```python
from build123d import *

# Parameters (mm, degrees)
F1_DEPTH     = 4.318
F1_FACE_W    = 8.4660017827
F1_FACE_H    = 4.318
F4_W         = 8.4660017827
F4_H         = 4.318
F5_DEPTH     = 0.508
F7_DEPTH     = 13.462
F9_T1_DEPTH  = 101.8009504956
F10_T1_DEPTH = 101.8156278686
F8_FACE_W    = 35.3900017827
F8_FACE_H    = 4.318
F14_DEPTH    = 45.466


# Not quite as in the source:
# - a fillet or chamfer that OpenCascade refuses, or shapes differently, is made with other operations: its cross-section is extruded or revolved along the edge and cut away or added


with BuildPart() as f1:
    # F0 (on Front) → F1 (new body)
    with BuildSketch(Plane.XZ):
        with BuildLine():
            ThreePointArc((-14.8547158409, -68.6793103814), (-12.973951869, -74.217922925), (-7.62, -76.5734910965))
            Line((-7.62, -76.5734910965), (7.62, -76.5734910965))
            ThreePointArc((7.62, -76.5734910965), (12.9819628095, -74.2196084737), (14.8784083325, -68.6793103814))
            Line((14.8784083325, -68.6793103814), (14.8547158409, -68.6793103814))
            Line((14.8547158409, -68.6793103814), (-14.8547158409, -68.6793103814))
        make_face()
        Polygon((-7.1831139455, 19.1512540919), (-14.8547158409, -68.6793103814), (14.8547158409, -68.6793103814), (7.1831139455, 19.1512540919), (4.2330008913, 52.9264810056), (-4.2330008913, 52.9264810056), align=None)
    extrude(amount=F1_DEPTH)

    # F3: sweep along a path in F2
    with BuildLine(Plane.YZ) as f3_path:
        Line((-4.318, 52.9264810056), (-4.318, 55.3578620488))
        ThreePointArc((-4.318, 55.3578620488), (-3.7519884271, 59.1070386053), (-2.1044055351, 62.5220297571))
        ThreePointArc((-2.1044055351, 62.5220297571), (2.3667917296, 72.1058812805), (3.5367051605, 82.6165005565))
    # F1_face (on face) → F3 (sweep)
    with BuildSketch(Plane(origin=(0, -2.159, 52.9264810056), x_dir=(1, 0, 0), z_dir=(0, 0, 1))):
        Rectangle(F1_FACE_W, F1_FACE_H)
    sweep(path=f3_path.line)

    # F4 (on face) → F5 (join)
    with BuildSketch(Plane(origin=(0, -4.2773000259, 82.2099457989), x_dir=(1, 0, 0), z_dir=(0, -0.0519587059, 0.9986492342))):
        with Locations((0, 9.9835743541)):
            Rectangle(F4_W, F4_H)
    extrude(amount=F5_DEPTH)

    # F6 (on face) → F7 (join)
    with BuildSketch(Plane.YZ.offset(4.2330008913)):
        with BuildLine():
            Line((-4.318, 52.9264810056), (0, 52.9264810056))
            Line((0, 52.9264810056), (0, 55.3578620488))
            ThreePointArc((0, 55.3578620488), (0.3735676381, 57.8323185761), (1.4609723468, 60.0862127363))
            ThreePointArc((1.4609723468, 60.0862127363), (6.5240819847, 70.938807275), (7.8488725536, 82.8408582485))
            Line((7.8488725536, 82.8408582485), (7.822477531, 83.3481720595))
            Line((7.822477531, 83.3481720595), (3.5103101379, 83.1238143674))
            Line((3.5103101379, 83.1238143674), (3.5367051605, 82.6165005565))
            ThreePointArc((3.5367051605, 82.6165005565), (2.3667917296, 72.1058812805), (-2.1044055351, 62.5220297571))
            ThreePointArc((-2.1044055351, 62.5220297571), (-3.7519884271, 59.1070386053), (-4.318, 55.3578620488))
            Line((-4.318, 55.3578620488), (-4.318, 52.9264810056))
        make_face()
    extrude(amount=F7_DEPTH)

    # F8: F1 across plane


with BuildPart() as f1_1:
    add(f1.part)
    add(f1.part.mirror(Plane.YZ))

    # F9: fillet of radius 20.8491483247 on 1 edges, made by hand

    # F9_s2 → F9_t1 (cut)
    with BuildSketch(Plane.XZ.offset(-48.7414752478)):
        with BuildLine():
            ThreePointArc((17.6950008913, 72.4230711047), (14.0025238199, 60.5767376056), (4.2330008913, 52.9264810056))
            Line((4.2330008913, 52.9264810056), (17.6950008913, 52.9264810056))
            Line((17.6950008913, 52.9264810056), (17.6950008913, 72.4230711047))
        make_face()
    extrude(amount=F9_T1_DEPTH, mode=Mode.SUBTRACT)

    # F10: fillet of radius 20.8534 on 1 edges, made by hand

    # F10_s2 → F10_t1 (cut)
    with BuildSketch(Plane.XZ.offset(-48.7488139343)):
        with BuildLine():
            ThreePointArc((-4.2330008913, 52.9264810056), (-14.0026048293, 60.5784652564), (-17.6950008913, 72.4260065793))
            Line((-17.6950008913, 72.4260065793), (-17.6950008913, 52.9264810056))
            Line((-17.6950008913, 52.9264810056), (-4.2330008913, 52.9264810056))
        make_face()
    extrude(amount=F10_T1_DEPTH, mode=Mode.SUBTRACT)

    # F12: sweep along a path in F11
    with BuildLine(Plane.YZ) as f12_path:
        ThreePointArc((5.6663938345, 83.2359932134), (4.2906494395, 90.7738508992), (1.2476332355, 97.8060641719))
        Line((1.2476332355, 97.8060641719), (-17.8702931298, 131.016411811))
    # F8_face (on face) → F12 (sweep)
    with BuildSketch(Plane(origin=(0, 5.6663938345, 83.2359932134), x_dir=(1, 0, 0), z_dir=(0, -0.0519587059, 0.9986492342))):
        Rectangle(F8_FACE_W, F8_FACE_H)
    sweep(path=f12_path.line)

    # F13 (on face) → F14 (cut)
    with BuildSketch(Plane(origin=(0, 41.3553334691, 23.8066830455), x_dir=(1, 0, 0), z_dir=(0, -0.8666583712, -0.4989020622))):
        Polygon((-6.7998209327, 122.4935306315), (-14.8516167313, 122.4935306315), (-11.232118832, 81.1224803329), (-10.419318832, 81.1224803329), align=None)
        Polygon((4.0258978993, 122.4935306315), (-4.0258978993, 122.4935306315), (-0.4064, 81.1224803329), (0, 81.1224803329), (0.4064, 81.1224803329), align=None)
        Polygon((11.232118832, 81.1224803329), (14.8516167313, 122.4935306315), (6.7998209327, 122.4935306315), (10.419318832, 81.1224803329), align=None)
    extrude(amount=-F14_DEPTH, mode=Mode.SUBTRACT)


solid = f1_1.part
```
CAD build for the part. Positions are in the model's coordinates, mm. A direction names the side the tool comes from. Round coordinates to 2 decimals unless told otherwise and drop trailing zeros. Order: outer loops, then holes, each group sorted by start corner. A loop starts at its lowest first (then second) coordinate and runs counter-clockwise, first axis right, second up. Notation, with made-up numbers: (19.5, 5) - (52.5, 5) arc R12 cw to (52.5, 10) - close; hole circle Ø4 at (89, 89.25). An arc over 180 degrees is marked (long way). Answer in a Markdown table with one row per item. Add a question column.
(1) Mould opens along X. For faces 1 (the face through (-8.635, -7.448, 112.85)), 2 (the face through (-12.925, -2.129, -74.281)), 3 (the face through (-15.329, -8.208, 109.904)) say: +X half, -X half, draft (parallel to the pull), parting line (faces both ways), or undercut.
(2) Probe L1, parallel to Y at x = -2, z = 38.5; L2, parallel to Z at x = 3, y = -2.25; L3, parallel to X at y = -1.75, z = -19. List the from-to ranges inside material, lowest first. Write a range as [from, to].
(3) Band-saw the part on B-B on y = -6.25. List the corners of the cut face in (x, z) (3 decimals).
(4) Band-saw the part on C-C on z = 67. List the corners of the cut face in (x, y), and give its area (3 significant figures).
(5) Band-saw the part on A-A on z = 107. List the corners of the cut face in (x, y) (3 decimals).
(6) Band-saw the part on D-D on z = -40. List the corners of the cut face in (x, y).
(7) Drop flat-ended pins along their axis: pin 1 Ø12 at (x, y) = (3.5, -4) entering from +Z; pin 2 Ø8 at (x, z) = (13.5, 18.5) entering from +Y; pin 3 Ø4 at (y, z) = (-3.5, -33) entering from -X; pin 4 Ø4 at (y, z) = (2.5, 69) entering from +X. Give the stop position or say it passes through.
(8) 3-axis set-ups, long thin cutter, end or side, ignore diameter. For faces 4 (the face through (14.1, 0.13, 60.72)), 5 (the face through (0, 0, -26)), 6 (the face through (15.242, -8.208, 109.904)): which of +Z, -Z, +X, -X, +Y, -Y reach the whole face in a straight line?
Data:
| question | item | result |
|---|---|---|
| 1 | face 1 | undercut |
| 1 | face 2 | -X half |
| 1 | face 3 | draft |
| 2 | L1 | y = [-4.32, 0] |
| 2 | L2 | z = [-76.57, 62.3], [99.55, 108.21] |
| 2 | L3 | x = [-10.52, 10.52] |
| 3 | outline | (-17.695, 106.503) - (-12.483, 106.503) - (-13.139, 115.157) - (-17.695, 115.157) - close; (-9.168, 106.503) - (-1.657, 106.503) - (-2.313, 115.157) - (-8.512, 115.157) - close; (1.657, 106.503) - (9.168, 106.503) - (8.512, 115.157) - (2.313, 115.157) - close; (12.483, 106.503) - (17.695, 106.503) - (17.695, 115.157) - (13.139, 115.157) - close |
| 4 | outline | (-16.98, 0.46) - (16.98, 0.46) - (16.98, 5.17) - (-16.98, 5.17) - close |
| 4 | area | 160 mm^2 |
| 5 | outline | (-17.695, -6.536) - (-12.533, -6.536) - (-12.316, -1.554) - (-17.695, -1.554) - close; (-9.336, -1.554) - (-9.118, -6.536) - (-1.707, -6.536) - (-1.49, -1.554) - close; (1.49, -1.554) - (1.707, -6.536) - (9.118, -6.536) - (9.336, -1.554) - close; (12.316, -1.554) - (12.533, -6.536) - (17.695, -6.536) - (17.695, -1.554) - close |
| 6 | outline | (-12.35, -4.32) - (12.35, -4.32) - (12.35, 0) - (-12.35, 0) - close |
| 7 | pin 1 | stops at z = 121.67 |
| 7 | pin 2 | passes through |
| 7 | pin 3 | stops at x = -11.91 |
| 7 | pin 4 | stops at x = 17.65 |
| 8 | face 4 | +X, +Y, -Y |
| 8 | face 5 | -Z, +X, -X, +Y |
| 8 | face 6 | +X, -X, -Y |
